Can you work these out from the model? Positions are in its coordinate system, mm. A direction names the side the tool comes from. Give positions to 0.01 mm unless a question says otherwise; leave off trailing zeros. Loops run counter-clockwise (first coordinate to the right, second up) from the corner with the lowest first, then second, coordinate; pieces in that order, holes last. Notation, with made-up numbers: (81.5, 84) -> (121.5, 84) arc R19 ccw to (121.5, 121) -> close; hole circle Ø6 at (33.25, 10.5). An arc over 180 degrees is marked (long way). Return JSON: item names as keys, results as strings. Group by question number.
Q1. Suppose I cut it at C-C, the plane y = 23. Please give me the cut outline in (x, z).
Q2. Will these pins go through, and if not, where does the flat tip stop? pin 1 (5 mm diameter, centred on x = 49.5, z = -40.5, fed in from +Y); pin 2 (5 mm diameter, centred on y = 40.25, z = -28.69, fed in from +X); pin 3 (5.5 mm diameter, centred on y = 69.5, z = -11.8, fed in from +X).
Q3. Which directions (+Z, -Z, +X, -X, +Y, -Y) give clear straight access to the entire face, cutting with the end or side of a thin tool? Please do faces 5 (the cylindrical face through (83.053, 57.887, 4.117)), 6 (the cylindrical face through (83.958, 30.427, -0.006)), 7 (the flat face through (43, 6, -24)).
Q4. I need wall thicknesses on line 1 along X through (y, z) = (15.5, -24); line 2 along X through (y, z) = (4, -23); line 3 along Z through (x, y) = (85.55, 20). Which ranges of each line are inside material? Lowest first, please. Write a range as [from, to].
Q5. Suppose I cut it at B-B, the plane z = -54. Please give me the cut outline in (x, y).
Q6. Suppose I cut it at A-A, the plane x = 43.5. Please give me the cut outline in (y, z) (3 decimals), and give its area (3 significant figures).
Q7. Suppose I cut it at D-D, the plane y = 50. Please give me the cut outline in (x, z).
Q8. Thinking about a two-plate mould opening in X: for faces 1 (the flat face through (44, 3, -26.95)), 2 (the cylindrical face through (83.053, 38.387, 4.117)), 3 (the flat face through (0, 34, -24)), 4 (the flat face through (6, 36, -24)), which applies, pulls with the +X half, pulls with the -X half, needs draft (parallel to the pull), parting line crosses it, or undercut?
```python
from build123d import *

# Parameters (mm, degrees)
SKETCH_1_W                   = 87
SKETCH_1_H                   = 60
SKETCH_1_R                   = 1.6
SKETCH_1_R_2                 = 2.025
EXTRUDE_1_DEPTH              = 6
SKETCH_2_R                   = 10
SKETCH_2_R_2                 = 2.05
EXTRUDE_2_DEPTH              = 6
FILLET_1_R                   = 20
FILLET_3_R                   = 5
FILLET_4_R                   = 10
FILLET_5_R                   = 10
HOLE_START                   = 81
HOLE_WIZARD_M3_1_OUTLINE_R   = 1.25
HOLE_WIZARD_M3_1_DEPTH       = 6
HOLE_WIZARD_M4_1_D           = 4.2
HOLE_WIZARD_M4_1_CSINK_D     = 8.1
HOLE_WIZARD_M4_1_CSINK_ANGLE = 90
HOLE_WIZARD_M4_2_D           = 4.2
HOLE_WIZARD_M4_2_CSINK_D     = 8.1
HOLE_WIZARD_M4_2_CSINK_ANGLE = 90


# Read off the part's stored shape, not the designer's step: M3 螺纹孔1
with BuildPart() as part:
    # 草图1 → 凸台-拉伸1 (new body)
    with BuildSketch(Plane(origin=(0, 0, 0), x_dir=(1, 0, 0), z_dir=(0, 1, 0))):
        with Locations((43.5, 30)):
            Rectangle(SKETCH_1_W, SKETCH_1_H)
        with Locations(Location((43.5, 43.5, 0), (0, 0, 270))):
            Circle(SKETCH_1_R, mode=Mode.SUBTRACT)
        with Locations(Location((55.191342951, 23.25, 0), (0, 0, 270))):
            Circle(SKETCH_1_R, mode=Mode.SUBTRACT)
        with Locations(Location((31.808657049, 23.25, 0), (0, 0, 270))):
            Circle(SKETCH_1_R, mode=Mode.SUBTRACT)
        with Locations(Location((54.022208656, 36.075, 0), (0, 0, 270))):
            Circle(SKETCH_1_R_2, mode=Mode.SUBTRACT)
        with Locations(Location((43.5, 17.85, 0), (0, 0, 270))):
            Circle(SKETCH_1_R_2, mode=Mode.SUBTRACT)
        with Locations(Location((32.977791344, 36.075, 0), (0, 0, 270))):
            Circle(SKETCH_1_R_2, mode=Mode.SUBTRACT)
        with BuildLine():
            Line((36.55, 33.05), (50.45, 33.05))
            ThreePointArc((50.45, 33.05), (51.864213562, 32.464213562), (52.45, 31.05))
            Line((52.45, 31.05), (52.45, 28.95))
            ThreePointArc((52.45, 28.95), (51.864213562, 27.535786438), (50.45, 26.95))
            Line((50.45, 26.95), (36.55, 26.95))
            ThreePointArc((36.55, 26.95), (35.135786438, 27.535786438), (34.55, 28.95))
            Line((34.55, 28.95), (34.55, 31.05))
            ThreePointArc((34.55, 31.05), (35.135786438, 32.464213562), (36.55, 33.05))
        make_face(mode=Mode.SUBTRACT)
    extrude(amount=EXTRUDE_1_DEPTH)

    # 草图2 → 凸台-拉伸2 (add)
    with BuildSketch(Plane(origin=(87, 0, 0), x_dir=(0, 0, -1), z_dir=(1, 0, 0))):
        with BuildLine():
            Line((60, 0), (60, 25))
            Line((60, 25), (30.584528933, 64.122584185))
            ThreePointArc((30.584528933, 64.122584185), (0.441305267, 70.571734049), (-10.155502807, 41.625004949))
            Line((-10.155502807, 41.625004949), (0, 15))
            Line((0, 15), (0, 0))
            Line((0, 0), (60, 0))
        make_face()
        with Locations((11.801488287, 50)):
            Circle(SKETCH_2_R, mode=Mode.SUBTRACT)
        with Locations((11.801488287, 69.5)):
            Circle(SKETCH_2_R_2, mode=Mode.SUBTRACT)
        with Locations((28.68898366, 59.75)):
            Circle(SKETCH_2_R_2, mode=Mode.SUBTRACT)
        with Locations((28.68898366, 40.25)):
            Circle(SKETCH_2_R_2, mode=Mode.SUBTRACT)
        with Locations((11.801488287, 30.5)):
            Circle(SKETCH_2_R_2, mode=Mode.SUBTRACT)
        with Locations((-5.086007087, 40.25)):
            Circle(SKETCH_2_R_2, mode=Mode.SUBTRACT)
        with Locations((-5.086007087, 59.75)):
            Circle(SKETCH_2_R_2, mode=Mode.SUBTRACT)
    extrude_2 = extrude(amount=-EXTRUDE_2_DEPTH)

    # 镜向1: 凸台-拉伸2 across plane
    add(extrude_2.mirror(Plane(origin=(43.5, 0, 0), x_dir=(0, 0, 1), z_dir=(1, 0, 0))))

    # 圆角1
    fillet_1_edges = [part.edges().sort_by_distance(p)[0] for p in [
        (3, 25, -60),
        (84, 25, -60),
    ]]
    fillet(fillet_1_edges, radius=FILLET_1_R)

    # 圆角3
    fillet_3_edges = [part.edges().sort_by_distance(p)[0] for p in [
        (6, 6, -30),
        (81, 6, -30),
    ]]
    fillet(fillet_3_edges, radius=FILLET_3_R)

    # 圆角4
    fillet_4_edges = [part.edges().sort_by_distance(p)[0] for p in [
        (87, 0, -30),
        (0, 0, -30),
    ]]
    fillet(fillet_4_edges, radius=FILLET_4_R)

    # 圆角5
    fillet_5_edges = [part.edges().sort_by_distance(p)[0] for p in [
        (3, 15, 0),
        (84, 15, 0),
    ]]
    fillet(fillet_5_edges, radius=FILLET_5_R)

    # Hole Wizard M3 _1 outline → Hole Wizard M3 _1 (cut)
    with BuildSketch(Plane.YZ.offset(HOLE_START)):
        with Locations((20, -6)):
            Circle(HOLE_WIZARD_M3_1_OUTLINE_R)
        with Locations((42.717410522, -39.171869507)):
            Circle(HOLE_WIZARD_M3_1_OUTLINE_R)
        with Locations((20, -45)):
            Circle(HOLE_WIZARD_M3_1_OUTLINE_R)
        with Locations((31.676227091, -0.060877223)):
            Circle(HOLE_WIZARD_M3_1_OUTLINE_R)
    extrude(amount=HOLE_WIZARD_M3_1_DEPTH, mode=Mode.SUBTRACT)

    # M4 十字槽半沉头木螺钉的锥形沉头孔1 (through all)
    with Locations(Plane.ZY):
        with Locations((-11.801488287, 69.5), (-28.68898366, 59.75), (-28.68898366, 40.25), (-11.801488287, 30.5), (5.086007087, 40.25), (5.086007087, 59.75)):
            CounterSinkHole(HOLE_WIZARD_M4_1_D / 2, HOLE_WIZARD_M4_1_CSINK_D / 2, counter_sink_angle=HOLE_WIZARD_M4_1_CSINK_ANGLE)

    # M4 十字槽半沉头木螺钉的锥形沉头孔2 (through all)
    with Locations(Plane(origin=(87, 0, 0), x_dir=(0, 0, -1), z_dir=(1, 0, 0))):
        with Locations((11.801488287, 69.5), (-5.086007087, 59.75), (-5.086007087, 40.25), (11.801488287, 30.5), (28.68898366, 40.25), (28.68898366, 59.75)):
            CounterSinkHole(HOLE_WIZARD_M4_2_D / 2, HOLE_WIZARD_M4_2_CSINK_D / 2, counter_sink_angle=HOLE_WIZARD_M4_2_CSINK_ANGLE)


solid = part.part
```
Ans:
{
 "1": {"outline": "(0, -59.44) -> (6, -59.44) -> (6, 3.05) -> (0, 3.05) -> close; (81, -59.44) -> (87, -59.44) -> (87, 3.05) -> (81, 3.05) -> close"},
 "2": {"pin 1": "stops at y = 6", "pin 2": "stops at x = 85.45", "pin 3": "stops at x = 85.7"},
 "3": {"face 5": "+X, -X", "face 6": "+X", "face 7": "+Z, -Z, +Y"},
 "4": {"line 1": "x = [0, 6], [81, 87]", "line 2": "x = [2, 30.23], [33.39, 53.61], [56.77, 85]", "line 3": "z = [-59.93, -46.25], [-43.75, -7.25], [-4.75, 1.91]"},
 "5": {"outline": "(0, 10) arc R10 ccw to (10, 0) -> (77, 0) arc R10 ccw to (87, 10) -> (87, 32.98) -> (81, 32.98) -> (81, 11) arc R5 cw to (76, 6) -> (11, 6) arc R5 cw to (6, 11) -> (6, 32.98) -> (0, 32.98) -> close"},
 "6": {"outline": "(0, -60) -> (6, -60) -> (6, -45.1) -> (0, -45.1) -> close; (0, -41.9) -> (6, -41.9) -> (6, -33.05) -> (0, -33.05) -> close; (0, -26.95) -> (6, -26.95) -> (6, -19.875) -> (0, -19.875) -> close; (0, -15.825) -> (6, -15.825) -> (6, 0) -> (0, 0) -> close", "area": "280 mm^2"},
 "7": {"outline": "(0, -41.2) -> (6, -41.2) -> (6, -21.8) -> (0, -21.8) -> close; (0, -1.8) -> (6, -1.8) -> (6, 11.7) -> (0, 11.7) -> close; (81, -41.2) -> (87, -41.2) -> (87, -21.8) -> (81, -21.8) -> close; (81, -1.8) -> (87, -1.8) -> (87, 11.7) -> (81, 11.7) -> close"},
 "8": {"face 1": "undercut", "face 2": "needs draft", "face 3": "pulls with the -X half", "face 4": "undercut"}
}
